Part model, mm, in its own coordinate system. A direction names the side the tool comes from. Coordinates: 2 decimals unless noted, no trailing zeros. Loops run counter-clockwise (first coordinate to the right, second up) from the corner with the lowest first, then second, coordinate; pieces in that order, holes last. Notation, with made-up numbers: M -35.5,39 L 9.5,39 A20 ccw 9.5,53 Z; hole C 11,-10.75 d10. An arc over 180 degrees is marked long. Use a Markdown table: item, result. Add a question column.
1) Band-saw the part on B-B (x = 13). List the corners of the cut face in (y, z).
2) Wall check: probe 1 along Y at (x, z) = (-15, 5); probe 2 along Z at (x, y) = (-10.5, 9); probe 3 along X at (y, z) = (8.5, -2.75). Give the ranges that are in metal, low to high. Write a range as from..to.
3) Band-saw the part on C-C (y = 14). List the corners of the cut face in (x, z).
4) Pull direction X, two halves, no side cores. Call faces 1 (the cylindrical face through (10.633, -9.905, -9.812)), 2 (the flat face through (-10.514, 10.93, -0.13)), 3 (the flat face through (18, -4.965, 0)): released by +X, released by -X, zero draft, split by the parting line, or undercut.
5) Band-saw the part on D-D (x = -1). List the corners of the cut face in (y, z).
6) Tool access for faces 4 (the flat face through (11, -8, 8)), 5 (the flat face through (-17.5, -5.5, -0.1)), 6 (the flat face through (18, -4, 9.75)), 7 (the flat face through (15, 6, 0)): list every direction of +Z, -Z, +X, -X, +Y, -Y with a clear straight run to the whole face (end or side of a thin tool).
7) Band-saw the part on A-A (z = -4). List the corners of the cut face in (x, y), plus the area to 4 significant figures.
8) Pin check, flat tips, straight feed: pin 1 Ø1.5 at (x, z) = (-17, -3) entering from +Y; pin 2 Ø5.5 at (x, z) = (-0.5, -3.5) entering from -Y; pin 3 Ø5 at (x, z) = (-7.5, -7.5) entering from -Y. Stop position of each tip, or through.
Autodesk Inventor part; units mm, degrees
ref_plane "Work Plane1" through (-19, -6, 9.25) normal (-1, 0, 0) x (0, 0, 1)
ref_plane "Work Plane3" through (5.5, 6, 9.25) normal (1, 0, 0) x (0, 0, -1)
ref_plane "YZ Plane" through (0, 0, 0) normal (1, 0, 0) x (0, 1, 0)
sketch "Sketch1" plane through (0, 0, 0) normal (0, 0, 1) x (1, 0, 0)
  line L0 (17.5, -6) -> (-17.5, -6)
  line L1 (-17.5, -6) -> (-17.5, 6)
  line L2 (-17.5, 6) -> (17.5, 6)
  line L3 (17.5, 6) -> (17.5, -6)
  line L4 (17.5, -6) -> (-17.5, 6) construction
  line L5 (-17.5, -6) -> (17.5, 6) construction
  line L6 (-11.5, 6) -> (-9.5, 16)
  line L7 (-9.5, 16) -> (6.5, 16)
  line L8 (6.5, 16) -> (12.5, 6)
  point P0 (0, 0)
  dimension "d0" = 35
  dimension "d1" = 12
  dimension "d2" = 16
  dimension "d3" = 6
  dimension "d4" = 5
  dimension "d5" = 11
  dimension "d6" = 16
extrude "Extrusion1" add sketch "Sketch1" along normal mid plane 18.5
sketch "Sketch2" plane through (0, 0, 0) normal (0, 0, 1) x (1, 0, 0)
  line L0 (17.5, -6) -> (-17.5, -6)
  circle A0 centre (-11.5, -6) radius 4
  circle A1 centre (11.5, -6) radius 4
  line L1 (17.5, -6) -> (17.5, 6)
  point P0 (0, 0)
  dimension "d9" = 8
  dimension "d10" = 8
  dimension "d11" = 6
  dimension "d12" = 23
extrude "Extrusion2" add sketch "Sketch2" along normal mid plane 22
sketch "Sketch3" plane through (-17.5, -6, 9.25) normal (-1, 0, 0) x (0, 0, 1)
  line L0 (-17.25, 0) -> (-1.25, 0)
  line L1 (-1.25, 0) -> (-1.25, -5.8773)
  line L2 (-1.25, -5.8773) -> (-17.25, -5.8773)
  line L3 (-17.25, -5.8773) -> (-17.25, 0)
  line L4 (1.75, -4) -> (1.75, 4)
  line L5 (0, 0) -> (-18.5, 0)
  point P0 (-9.25, 6)
  dimension "d15" = 16
  dimension "d16" = 3
extrude "Extrusion3" cut sketch "Sketch3" against normal blind 35
ref_plane "Work Plane1" through (-19, -6, 9.25) normal (-1, 0, 0) x (0, 0, 1)
sketch "Sketch4" plane through (-19, -6, 9.25) normal (-1, 0, 0) x (0, 0, 1)
  line L0 (-19, 3.5348) -> (0.5, 3.5348)
  line L1 (0.5, 3.5348) -> (0.5, 1.0348)
  line L2 (0.5, 1.0348) -> (-19, 1.0348)
  line L3 (-19, 1.0348) -> (-19, 3.5348)
  line L4 (0, 12) -> (0, 0)
  point P0 (-9.25, 6)
  dimension "d20" = 2.5
  dimension "d21" = 19.5
  dimension "d22" = 0.5
extrude "Extrusion4" add sketch "Sketch4" against normal blind 3
mirror "Mirror1" about plane through (0, 0, 0) normal (1, 0, 0) of "Extrusion4"
ref_plane "Work Plane3" through (5.5, 6, 9.25) normal (1, 0, 0) x (0, 0, -1)
sketch "Sketch5" plane through (5.5, 6, 9.25) normal (1, 0, 0) x (0, 0, -1)
  line L0 (1.25, -16) -> (-1.75, -16)
  line L1 (20.25, -16) -> (17.25, -16)
  circle A0 centre (9.25, -16) radius 2.5
  point P0 (9.25, -6)
  dimension "d26" = 5
boundary_patch "Boundary Patch1"
properties part number "Car"
Entries:
| question | item | result |
|---|---|---|
| 1 | outline | M -9.71,-11 L -2.29,-11 L -2.29,-9.25 L 6,-9.25 L 6,9.25 L -2.29,9.25 L -2.29,11 L -9.71,11 L -9.71,8 L -6,8 L -6,-8 L -9.71,-8 Z |
| 2 | probe 1 | -6..6 |
| 2 | probe 2 | -9.25..9.25 |
| 2 | probe 3 | -11..11 |
| 3 | outline | M -9.9,-9.25 L 7.7,-9.25 L 7.7,9.25 L -9.9,9.25 Z |
| 4 | face 1 | undercut |
| 4 | face 2 | released by -X |
| 4 | face 3 | zero draft |
| 5 | outline | M -6,-9.25 L 16,-9.25 L 16,9.25 L -6,9.25 Z |
| 6 | face 4 | +X, -X, -Y |
| 6 | face 5 | +Z, -Z, -X, -Y |
| 6 | face 6 | +Z, +X, +Y, -Y |
| 6 | face 7 | +Z, -Z, +X, +Y |
| 7 | outline | M -19,-4.97 L -17.5,-4.97 L -17.5,-6 L 17.5,-6 L 17.5,-4.97 L 19,-4.97 L 19,-2.47 L 17.5,-2.47 L 17.5,6 L 12.5,6 L 6.5,16 L -9.5,16 L -11.5,6 L -17.5,6 L -17.5,-2.47 L -19,-2.47 Z |
| 7 | area | 627.5 mm2 |
| 8 | pin 1 | y = 6 |
| 8 | pin 2 | y = -6 |
| 8 | pin 3 | y = -9.69 |
